Check sheet for the modelled part. Datum: model origin and axes. Units: mm. Face numbers are marked on the shaded views. A direction names the side the tool comes from. Round coordinates to 2 decimals unless told otherwise and drop trailing zeros. Order: outer loops, then holes, each group sorted by start corner. A loop starts at its lowest first (then second) coordinate and runs counter-clockwise, first axis right, second up.
```python
from build123d import *

# Parameters (mm, degrees)
F0_R     = 2.1463
F1_DEPTH = 5.08


with BuildPart() as f1:
    # F0 (on Front) → F1 (new body)
    with BuildSketch(Plane.XZ):
        with BuildLine():
            Line((6.35, -4.7625), (6.35, 4.7625))
            Line((6.35, 4.7625), (4.826, 4.7625))
            Line((4.826, 4.7625), (0, -0.0635))
            Line((0, -0.0635), (-4.826, 4.7625))
            Line((-4.826, 4.7625), (-6.35, 4.7625))
            Line((-6.35, 4.7625), (-6.35, -4.7625))
            ThreePointArc((-6.35, -4.7625), (0, -11.1125), (6.35, -4.7625))
        make_face()
        with Locations((0, -4.7625)):
            Circle(F0_R, mode=Mode.SUBTRACT)
    extrude(amount=F1_DEPTH)


solid = f1.part
```
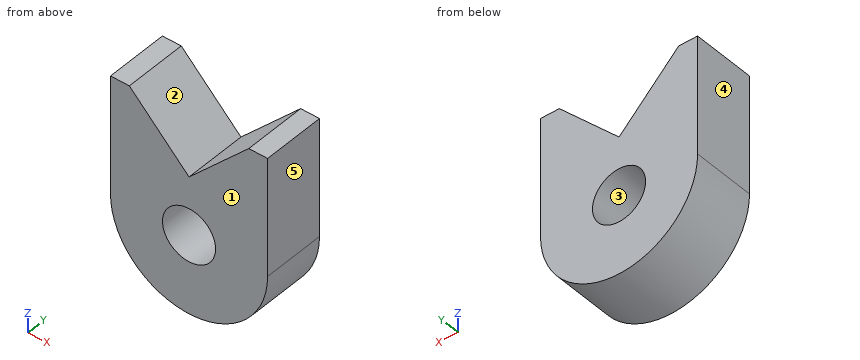
Item 1: Sectioned sample at C-C (z = 3.25). Record the cut outline in (x, y), and give its area (3 significant figures).
Answer:
outline: (-6.35, -5.08) - (-3.31, -5.08) - (-3.31, 0) - (-6.35, 0) - close; (3.31, -5.08) - (6.35, -5.08) - (6.35, 0) - (3.31, 0) - close
area: 30.9 mm2
Item 2: Access from +Z, -Z, +X, -X, +Y, -Y to the whole of each face (thin tool, end or side, straight path). Record for the marked faces 1 and 2.
Answer:
face 1: +Z, -Z, +X, -X, -Y
face 2: +Z, +Y, -Y
Item 3: Scan lines: line 1 along X through (y, z) = (-2.05, 1.5); line 2 along X through (y, z) = (-3.05, 0.25); line 3 along Z through (x, y) = (4, -2.55). Record each from-to range of solid material in increasing order.
Answer:
line 1: x = -6.35 to -1.56, 1.56 to 6.35
line 2: x = -6.35 to -0.31, 0.31 to 6.35
line 3: z = -9.69 to 3.94
Item 4: Sectioned sample at A-A (y = -4.05). Record the cut outline in (x, z), and give its area (3 significant figures).
Answer:
outline: (-6.35, -4.76) arc R6.35 ccw to (6.35, -4.76) - (6.35, 4.76) - (4.83, 4.76) - (0, -0.06) - (-4.83, 4.76) - (-6.35, 4.76) - close; hole circle Ø4.29 at (0, -4.76)
area: 147 mm2
Item 5: Release check for a two-part mould opening along X. For the marked faces 3, 4 and 5 record: released by +X, released by -X, zero draft, split by the parting line, or undercut.
Answer:
face 3: undercut
face 4: released by -X
face 5: released by +X
Item 6: Sectioned sample at B-B (x = 0.25). Record the cut outline in (y, z), and give its area (3 significant figures).
Answer:
outline: (-5.08, -11.11) - (0, -11.11) - (0, -6.89) - (-5.08, -6.89) - close; (-5.08, -2.63) - (0, -2.63) - (0, 0.19) - (-5.08, 0.19) - close
area: 35.7 mm2
Item 7: Sectioned sample at D-D (z = -10). Record the cut outline in (x, y).
Answer:
outline: (-3.59, -5.08) - (3.59, -5.08) - (3.59, 0) - (-3.59, 0) - close
